from build123d import *

# Parameters (mm, degrees)
SKETCH_R        = 12
PAD_DEPTH       = 7.8
SKETCH001_R     = 12
SKETCH001_R_2   = 10.4
SKETCH001_R_3   = 1.15
PAD001_DEPTH    = 5
SKETCH002_R     = 15
PAD002_DEPTH    = 40
PAD003_DEPTH    = 10
SKETCH004_R     = 1.65
POCKET_DEPTH    = 52.801
SKETCH005_R     = 4
POCKET001_DEPTH = 37.8


with BuildPart() as part:
    # Sketch → Pad (new body)
    with BuildSketch(Plane.XZ):
        Circle(SKETCH_R)
    extrude(amount=PAD_DEPTH)

    # Sketch001 (on Face2 of Pad) → Pad001 (join)
    with BuildSketch(Plane(origin=(0, 0, 0), x_dir=(1, 0, 0), z_dir=(0, 1, 0))):
        Circle(SKETCH001_R)
        Circle(SKETCH001_R_2, mode=Mode.SUBTRACT)
        with Locations((0, 7.3)):
            Circle(SKETCH001_R_3)
        with Locations((7.3, 0)):
            Circle(SKETCH001_R_3)
        with Locations((0, -7.3)):
            Circle(SKETCH001_R_3)
        with Locations((-7.3, 0)):
            Circle(SKETCH001_R_3)
    extrude(amount=PAD001_DEPTH)

    # Sketch002 (on Face1 of Pad001) → Pad002 (join)
    with BuildSketch(Plane.XZ.offset(7.8)):
        Circle(SKETCH002_R)
    extrude(amount=PAD002_DEPTH)

    # Sketch003 (on Face6 of Pad002) → Pad003 (join)
    with BuildSketch(Plane.XZ.offset(47.8)):
        with BuildLine():
            ThreePointArc((0, 15), (-15, 0), (0, -15))
            Line((0, -15), (90, -15))
            ThreePointArc((90, -15), (105, 0), (90, 15))
            Line((0, 15), (90, 15))
        make_face()
    extrude(amount=-PAD003_DEPTH)

    # Sketch004 (on Face5 of Pad003) → Pocket (cut, through all)
    with BuildSketch(Plane.XZ.offset(47.8)):
        Circle(SKETCH004_R)
    extrude(amount=-POCKET_DEPTH, mode=Mode.SUBTRACT)

    # Sketch005 (on Face6 of Pocket) → Pocket001 (cut)
    with BuildSketch(Plane.XZ.offset(47.8)):
        Circle(SKETCH005_R)
    extrude(amount=-POCKET001_DEPTH, mode=Mode.SUBTRACT)


solid = part.part
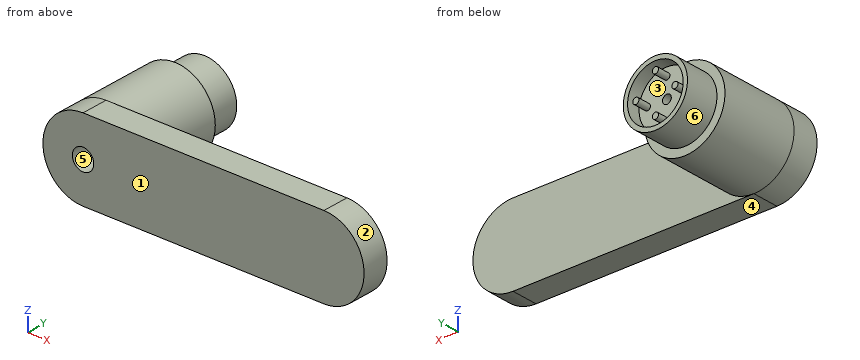
The listing builds one solid part. Answer for the finished solid, in the listing's coordinates (mm). Face numbers are marked on the shaded views. A direction names the side the tool comes from. Coordinates: 2 decimals unless noted, no trailing zeros. Order: outer loops, then holes, each group sorted by start corner. A loop starts at its lowest first (then second) coordinate and runs counter-clockwise, first axis right, second up. Notation, with made-up numbers: (87.5, 20) -> (99.5, 20) arc R29 ccw to (99.5, 50) -> close; hole circle Ø6 at (5.25, 43.5). An arc over 180 degrees is marked (long way). Answer in a Markdown table with one row per item. Add a question column.
Item 1: Find section B-B (y = -44). Write down the section's boundary in (x, z), then the cut area to 3 significant figures.
Item 2: Find section D-D (z = -7.3). Write down the section's boundary in (x, y).
Item 3: Determine the mould class of the marked faces 1, 2 and 3 for opening direction Z: +Z half, -Z half, draft (parallel to the pull), parting line (faces both ways), or undercut.
Item 4: Which of the six approach directions +Z, -Z, +X, -X, +Y, -Y give full straight-line access (tool end or side, diameter ignored) to the marked faces 4, 5 and 6?
Item 5: Find the intervals of material crossed by L1, parallel to X at y = 2, z = 0; L2, parallel to Z at x = 0, y = -21, in increasing order. Write a range as from..to.
Item 6: Each of these flat-tipped pins is pushed along its axis until it touches: P1, Ø6, axis at x = 72, z = 3, coming from the +Y side; P2, Ø1, axis at y = -35.5, z = -4, coming from the -X side; P3, Ø10, axis at y = -3.5, z = -1, coming from the -X side; P4, Ø6.5, axis at x = 0, z = 0, coming from the +Y side. Where does it stop, or does it pass through?
Item 7: Find section C-C (x = 26.5). Write down the section's boundary in (y, z), then the cut area to 3 significant figures.
Result set:
| question | item | result |
|---|---|---|
| 1 | outline | (0, -15) -> (90, -15) arc R15 ccw to (90, 15) -> (0, 15) arc R15 ccw to start; hole circle Ø8 at (0, 0) |
| 1 | area | 3,360 mm² |
| 2 | outline | (-13.1, -47.8) -> (103.1, -47.8) -> (103.1, -37.8) -> (13.1, -37.8) -> (13.1, -7.8) -> (9.52, -7.8) -> (9.52, 5) -> (7.41, 5) -> (7.41, 0) -> (1.15, 0) -> (1.15, 5) -> (-1.15, 5) -> (-1.15, 0) -> (-7.41, 0) -> (-7.41, 5) -> (-9.52, 5) -> (-9.52, -7.8) -> (-13.1, -7.8) -> close |
| 3 | face 1 | draft |
| 3 | face 2 | parting line |
| 3 | face 3 | undercut |
| 4 | face 4 | -Z, +X, -X, +Y, -Y |
| 4 | face 5 | -Y |
| 4 | face 6 | +Y |
| 5 | L1 | x = -12..-10.4, -8.45..-6.15, 6.15..8.45, 10.4..12 |
| 5 | L2 | z = -15..-4, 4..15 |
| 6 | P1 | stops at y = -37.8 |
| 6 | P2 | stops at x = -14.59 |
| 6 | P3 | stops at x = -15 |
| 6 | P4 | stops at y = 0 |
| 7 | outline | (-47.8, -15) -> (-37.8, -15) -> (-37.8, 15) -> (-47.8, 15) -> close |
| 7 | area | 300 mm² |
